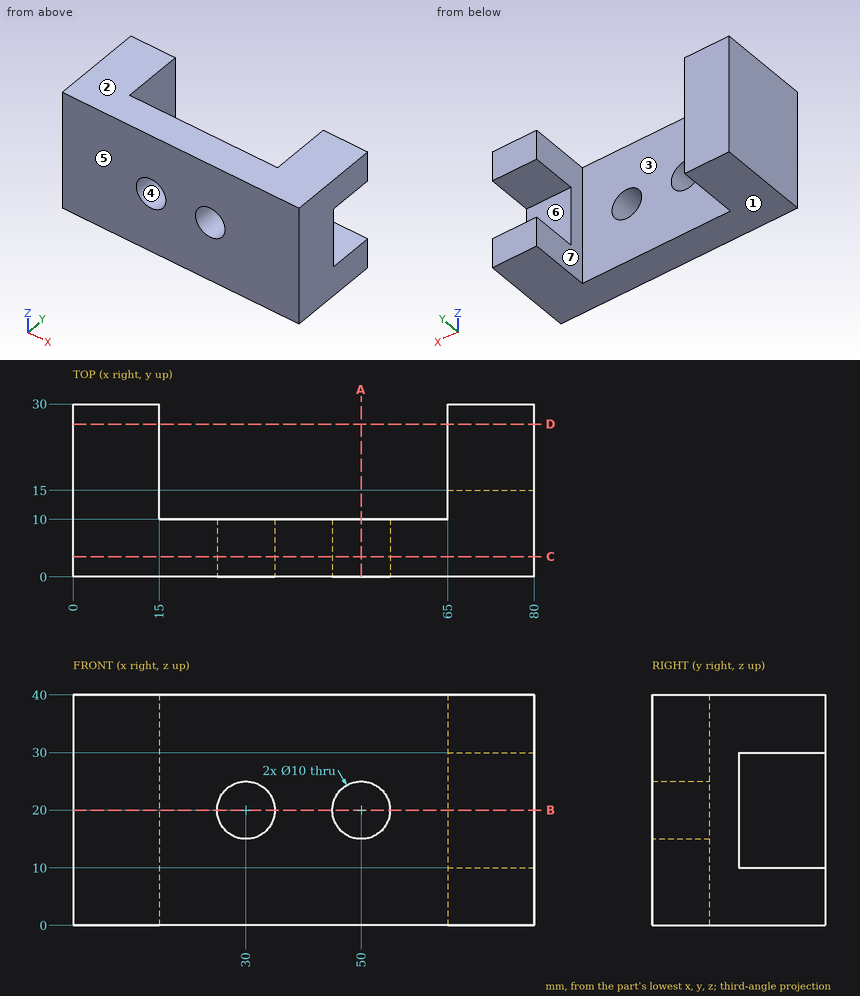
Design review of the part shown in the three views and the two pictorial views. Dimensions are in mm from the part's minimum x, y and z. A direction names the side the tool comes from. Round coordinates to 2 decimals unless told otherwise and drop trailing zeros. Loops run counter-clockwise (first coordinate to the right, second up) from the corner with the lowest first, then second, coordinate; pieces in that order, holes last. Notation, with made-up numbers: (-36.5, 38.5) -> (15.5, 38.5) arc R25 cw to (15.5, 54.5) -> close; hole circle Ø5 at (-18.5, 24). An arc over 180 degrees is marked (long way). Return JSON: item names as keys, results as strings.
(1) For the marked faces 5, 6 and 7, list the 3-axis set-ups (+Z, -Z, +X, -X, +Y, -Y) from which the entire face can be reached by the end or side of a thin tool; tool diameter is ignored.
Solved:
{"face 5": "+Z, -Z, +X, -X, -Y", "face 6": "+X, +Y", "face 7": "+Z, -Z, +Y"}
(2) Add section C-C on y = 3.5. Write out the cut boundary in (x, z).
Solved:
{"outline": "(0, 0) -> (80, 0) -> (80, 40) -> (0, 40) -> close; hole circle Ø10 at (30, 20); hole circle Ø10 at (50, 20)"}
(3) For pin 1 (2 mm diameter, centred on x = 56.5, z = 25, fed in from +Y); pin 2 (3 mm diameter, centred on x = 65, z = 17.5, fed in from +Y), all flat-tipped, find the tip position at first contact; note any pin that passes through.
Solved:
{"pin 1": "y = 10", "pin 2": "y = 15"}
(4) Add section D-D on y = 26.5. Write out the cut boundary in (x, z).
Solved:
{"outline": "(0, 0) -> (15, 0) -> (15, 40) -> (0, 40) -> close; (65, 0) -> (80, 0) -> (80, 10) -> (65, 10) -> close; (65, 30) -> (80, 30) -> (80, 40) -> (65, 40) -> close"}
(5) For line 1 (X direction, y = 6.75, z = 20); line 2 (X direction, y = 17.25, z = 38); line 3 (Y direction, x = 45, z = 7), list the stretches that pass through material, from the lowest coordinate up.
Solved:
{"line 1": "0 to 25, 35 to 45, 55 to 80", "line 2": "0 to 15, 65 to 80", "line 3": "0 to 10"}
(6) Add section B-B on z = 20. Write out the cut boundary in (x, y), plus the area to 3 significant figures.
Solved:
{"outline": "(0, 0) -> (25, 0) -> (25, 10) -> (15, 10) -> (15, 30) -> (0, 30) -> close; (35, 0) -> (45, 0) -> (45, 10) -> (35, 10) -> close; (55, 0) -> (80, 0) -> (80, 15) -> (65, 15) -> (65, 10) -> (55, 10) -> close", "area": "975 mm2"}
(7) Add section A-A on x = 50. Write out the cut boundary in (y, z), plus the area to 3 significant figures.
Solved:
{"outline": "(0, 0) -> (10, 0) -> (10, 15) -> (0, 15) -> close; (0, 25) -> (10, 25) -> (10, 40) -> (0, 40) -> close", "area": "300 mm2"}
(8) The part is to be moulded in two halves that separate along Z. For the marked faces 1, 2, 3 and 4, say which applies: released by +Z, released by -Z, zero draft, split by the parting line, or undercut.
Solved:
{"face 1": "released by -Z", "face 2": "released by +Z", "face 3": "zero draft", "face 4": "undercut"}
